Verification items for the finished model (mm, model axes). Round coordinates to 2 decimals unless told otherwise and drop trailing zeros. Order: outer loops, then holes, each group sorted by start corner. A loop starts at its lowest first (then second) coordinate and runs counter-clockwise, first axis right, second up. Notation, with made-up numbers: M 60.25,-34.75 L 69.25,-34.75 A26 cw 69.25,-13.75 Z; hole C 56,77 d8. An arc over 180 degrees is marked long. Use one line per item in the form item = value. Start each with the question number.
Item 1: Cross-section at C-C on z = 92. Enter the section's corners in (x, y).
Item 2: Go/stop test with flat-tipped pins: pin 1 Ø0.9 at (x, y) = (0.5, -7) entering from -Z; pin 2 Ø1.5 at (y, z) = (-9, 14.5) entering from -X; pin 3 Ø4 at (x, z) = (4.5, 45) entering from -Y. Record where each tip stops, or that it passes through.
Item 3: Cross-section at A-A on x = 0. Enter the section's corners in (y, z).
Item 4: Cross-section at B-B on y = 3.5. Enter the section's corners in (x, z), then the cut area to 3 significant figures.
Item 5: Thickness scan on probe 1 along X at (y, z) = (2, 56.5); probe 2 along Y at (x, z) = (-0.25, 33); probe 3 along X at (y, z) = (0.75, 90). Record the ranges inside material, lowest first. Write a range as [from, to].
Item 6: Cross-section at D-D on x = 6.25. Enter the section's corners in (y, z).
from build123d import *

# Parameters (mm, degrees)
BOSS_EXTRUDE1_DEPTH = 150
BOSS_EXTRUDE6_DEPTH = 1.5
SKETCH7_R           = 0.5
BOSS_EXTRUDE7_DEPTH = 4


with BuildPart() as part:
    # Sketch1 → Boss-Extrude1 (new body)
    with BuildSketch(Plane.XY):
        with BuildLine():
            Line((7.5, 5), (5, 5))
            ThreePointArc((5, 5), (0, 0), (-5, 5))
            Line((-5, 5), (-7.5, 5))
            Line((-7.5, 5), (-7.5, -5))
            Line((-7.5, -5), (7.5, -5))
            Line((7.5, -5), (7.5, 5))
        make_face()
    extrude(amount=BOSS_EXTRUDE1_DEPTH)

    # Sketch6 → Boss-Extrude6 (add, symmetric)
    with BuildSketch(Plane.ZY):
        with BuildLine():
            ThreePointArc((77.5, -8), (75, -5.5), (72.5, -8))
            Line((72.5, -8), (77.5, -8))
        make_face()
        with BuildLine():
            Line((77.5, -8), (72.5, -8))
            ThreePointArc((72.5, -8), (75, -10.5), (77.5, -8))
        make_face()
        with BuildLine():
            Line((77.5, -5), (72.5, -5))
            Line((72.5, -5), (72.5, -8))
            ThreePointArc((72.5, -8), (75, -5.5), (77.5, -8))
            Line((77.5, -8), (77.5, -5))
        make_face()
    boss_extrude6 = extrude(amount=BOSS_EXTRUDE6_DEPTH, both=True)

    # Sketch7 → Boss-Extrude7 (add, symmetric)
    with BuildSketch(Plane.ZY):
        with Locations((75, -8)):
            Circle(SKETCH7_R)
    boss_extrude7 = extrude(amount=BOSS_EXTRUDE7_DEPTH, both=True)

    # Mirror1: Boss-Extrude6 across plane
    add(boss_extrude6.mirror(Plane(origin=(0, 0, 45), x_dir=(1, 0, 0), z_dir=(0, 0, -1))))

    # Mirror2: Boss-Extrude7 across plane
    add(boss_extrude7.mirror(Plane(origin=(0, 0, 45), x_dir=(1, 0, 0), z_dir=(0, 0, -1))))


solid = part.part
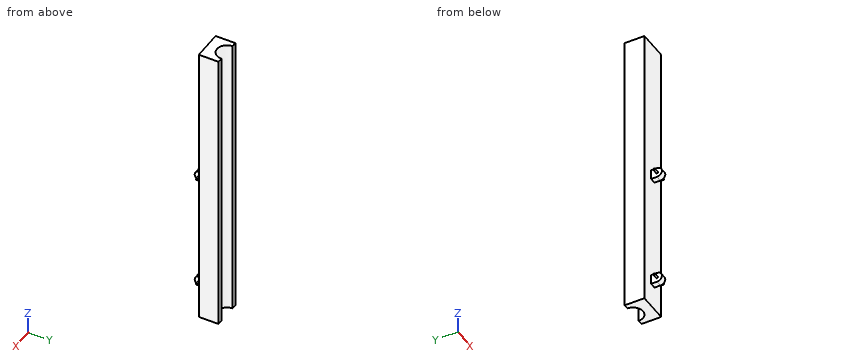
Output values:
q1.outline = M -7.5,-5 L 7.5,-5 L 7.5,5 L 5,5 A5 cw -5,5 L -7.5,5 Z
q2.pin_1 = 12.5
q2.pin_2 = -4
q2.pin_3 = -5
q3.outline = M -8,12.5 L -5,12.5 L -5,0 L 0,0 L 0,150 L -5,150 L -5,77.5 L -8,77.5 A2.5 ccw -8,72.5 L -5,72.5 L -5,17.5 L -8,17.5 A2.5 ccw Z
q4.outline = M -7.5,0 L -4.77,0 L -4.77,150 L -7.5,150 Z; M 4.77,0 L 7.5,0 L 7.5,150 L 4.77,150 Z
q4.area = 819 mm2
q5.probe_1 = [-7.5, -4], [4, 7.5]
q5.probe_2 = [-5, 0.01]
q5.probe_3 = [-7.5, -2.63], [2.63, 7.5]
q6.outline = M -5,0 L 5,0 L 5,150 L -5,150 Z
